Can you work these out from the model? Positions are in its coordinate system, mm. Coordinates: 2 decimals unless noted, no trailing zeros. Order: outer loops, then holes, each group sorted by start corner. A loop starts at its lowest first (then second) coordinate and runs counter-clockwise, first axis right, second up. Notation, with made-up numbers: M -17.5,-16.5 L 15.5,-16.5 A17 cw 15.5,1.5 Z; hole C 47,-38 d6. An arc over 180 degrees is marked long. Answer as a JSON object with one key per item and string values.
from build123d import *
from build123d.topology import SkipClean

# Parameters (mm, degrees)
BOSS_EXTRUDE1_DEPTH     = 1174.75
F_1_2_CLEARANCE_HOLE1_D = 13.09624
SKETCH116_R             = 25.146
SKETCH116_R_2           = 6.54812
BOSS_EXTRUDE2_DEPTH     = 4.953


with BuildPart() as part:
    # Sketch113 → Boss-Extrude1 (new body)
    with BuildSketch(Plane.XY):
        with BuildLine():
            Line((0, 0), (0, 49.2252))
            Line((0, 49.2252), (7.9248, 49.2252))
            Line((7.9248, 49.2252), (7.9248, 20.6248))
            ThreePointArc((7.9248, 20.6248), (11.644543879, 11.644543879), (20.6248, 7.9248))
            Line((20.6248, 7.9248), (55.5752, 7.9248))
            ThreePointArc((55.5752, 7.9248), (64.555456121, 11.644543879), (68.2752, 20.6248))
            Line((68.2752, 20.6248), (68.2752, 49.2252))
            Line((68.2752, 49.2252), (76.2, 49.2252))
            Line((76.2, 49.2252), (76.2, 0))
            Line((76.2, 0), (0, 0))
        make_face()
    extrude(amount=BOSS_EXTRUDE1_DEPTH)

    # 1_2 Clearance Hole1 (through all)
    with Locations(Plane(origin=(38.1, 0, 206.375), x_dir=(0, 0, -1), z_dir=(0, -1, 0))):
        with Locations((0, 0), (-762, 0)):
            Hole(F_1_2_CLEARANCE_HOLE1_D / 2)

    # Sketch116 → Boss-Extrude2 (add)
    # profile 1 of 2: a face of its own
    with SkipClean():  # the faces are left unmerged after this step: merging them gives an invalid solid
        with BuildSketch(Plane.XZ):
            with Locations(Location((38.1, 968.375, 0), (0, 0, 180))):
                Circle(SKETCH116_R)
            with Locations(Location((38.1, 968.375, 0), (0, 0, 270))):
                Circle(SKETCH116_R_2, mode=Mode.SUBTRACT)
        # profile 2 of 2: a face of its own
        with BuildSketch(Plane.XZ):
            with Locations(Location((38.1, 206.375, 0), (0, 0, 180))):
                Circle(SKETCH116_R)
            with Locations(Location((38.1, 206.375, 0), (0, 0, 270))):
                Circle(SKETCH116_R_2, mode=Mode.SUBTRACT)
        extrude(amount=BOSS_EXTRUDE2_DEPTH)
    add(part.part.scale(1), mode=Mode.REPLACE)  # the faces are merged on a copy


solid = part.part
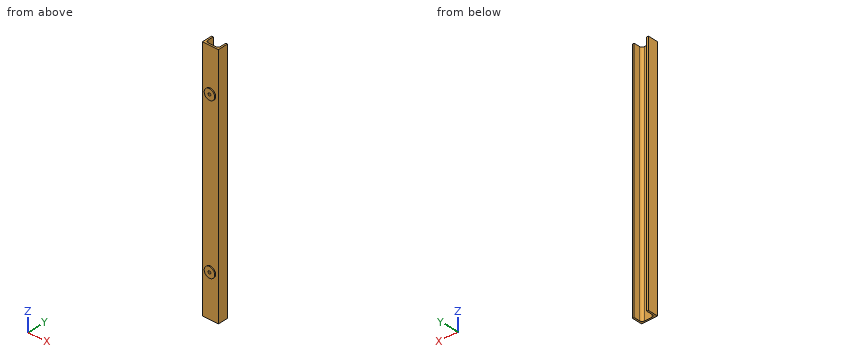
Item 1: Please list where these lines run through material, in increasing order: line 1 (Z direction, x = 38.1, y = -1.8); line 2 (Z direction, x = 38, y = 2); line 3 (X direction, y = 30.5, z = 834).
Answers follow:
{"line 1": "z = 181.23 to 199.83, 212.92 to 231.52, 943.23 to 961.83, 974.92 to 993.52", "line 2": "z = 0 to 199.83, 212.92 to 961.83, 974.92 to 1174.75", "line 3": "x = 0 to 7.92, 68.28 to 76.2"}
Item 2: I'm going to push flat-ended pins straight in: pin 1 (4 mm diameter, centred on x = 27, y = 10, fed in from -Z); pin 2 (15 mm diameter, centred on x = 38.1, z = 206.375, fed in from +Y). Where does each tip first touch, or does it pass through?
Answers follow:
{"pin 1": "passes through", "pin 2": "stops at y = 7.92"}
Item 3: I want a section at A-A, the plane y = 36.5. Write out the boundary of the cut face in (x, z), plus the area to 3 significant figures.
Answers follow:
{"outline": "M 0,0 L 7.92,0 L 7.92,1174.75 L 0,1174.75 Z; M 68.28,0 L 76.2,0 L 76.2,1174.75 L 68.28,1174.75 Z", "area": "18,600 mm^2"}
Item 4: I want a section at B-B, the plane z = 1021. Write out the boundary of the cut face in (x, y), plus the area to 3 significant figures.
Answers follow:
{"outline": "M 0,0 L 76.2,0 L 76.2,49.23 L 68.28,49.23 L 68.28,20.62 A12.7 cw 55.58,7.92 L 20.62,7.92 A12.7 cw 7.92,20.62 L 7.92,49.23 L 0,49.23 Z", "area": "1,330 mm^2"}
